Input: part model. Units: mm. Frame: model coordinates. A direction names the side the tool comes from. Round coordinates to 2 decimals unless told otherwise and drop trailing zeros. Loops run counter-clockwise (first coordinate to the right, second up) from the corner with the lowest first, then second, coordinate; pieces in that order, holes last. Notation, with made-up numbers: (-24.5, 70) -> (14.5, 70) arc R17 ccw to (14.5, 86) -> close; hole circle Ø5 at (45.25, 86.5). An arc over 180 degrees is marked (long way). One line per question, with ' | ' between items. Start each with the question number.
Q1. Cut plane B-B on z = 2.5. Return loops of the section in (x, y).
Q2. Access query for faces 1 (the face through (37, 44.45, 3)), 2 (the face through (-1.33, -5.59, 3.13)), 3 (the face through (0, 42, 3)). Directions: +Z, -Z, +X, -X, +Y, -Y. A direction counts if a zero-diameter tool reaches every point of the face in a straight line with its end or side. Return the directions, or none.
Q3. Cut plane D-D on y = 55. Return loops of the section in (x, z), and give its area (3 significant figures).
Q4. Material intervals for L1, parallel to X at y = 22.5, z = 4; L2, parallel to Y at x = 6.5, z = 6.25; L3, parallel to X at y = 52.5, z = 3, sorted ascending.
Q5. Cut plane C-C on x = 29. Return loops of the section in (y, z), and give its area (3 significant figures).
Q6. Contact query for flat-ended pins moving along their axis: P1, Ø3, axis at y = 46.5, z = 4, coming from the +X side; P2, Ø2, axis at x = 36, z = 4, coming from the +Y side; P3, Ø12, axis at x = 35.5, y = 43, coming from the -Z side; P4, Ø3, axis at x = 21.5, z = 2, coming from the +Y side. Output: stop coordinate, or through.
Q7. Cut plane A-A on y = 30.5. Return loops of the section in (x, z), and give its area (3 significant figures).
from build123d import *

# Parameters (mm, degrees)
BOSS_EXTRUDE1_DEPTH = 6.35
FILLET1_R           = 2.54


with BuildPart() as part:
    # Sketch1 → Boss-Extrude1 (new body)
    with BuildSketch(Plane.XY):
        Polygon((0, 0), (35.3568, 0), (35.3568, 44.45), (41.7068, 44.45), (41.7068, -6.35), (-2.0574, -6.35), (-2.0574, 82.55), (0, 82.55), align=None)
    extrude(amount=BOSS_EXTRUDE1_DEPTH)

    # Fillet1
    # the kernel refuses this fillet: 2.54 mm, written as the material it takes off along each edge
    with BuildSketch(Plane(origin=(41.7068, 44.45, -6.35), x_dir=(-1, 0, 0), z_dir=(0, 0, 1)), Plane(origin=(-2.0574, -6.35, -6.35), x_dir=(1, 0, 0), z_dir=(0, 0, 1)), Plane(origin=(41.7068, -6.35, -6.35), x_dir=(0, 1, 0), z_dir=(0, 0, 1))) as fillet1_piece_1:
        with BuildLine():
            CenterArc((FILLET1_R, FILLET1_R), FILLET1_R, 180, 90)
            Line((0, FILLET1_R), (-FILLET1_R * 0.02, FILLET1_R))
            Line((-FILLET1_R * 0.02, FILLET1_R), (-FILLET1_R * 0.02, -FILLET1_R * 0.02))
            Line((-FILLET1_R * 0.02, -FILLET1_R * 0.02), (FILLET1_R, -FILLET1_R * 0.02))
            Line((FILLET1_R, -FILLET1_R * 0.02), (FILLET1_R, 0))
        make_face()
    extrude(amount=19.05, mode=Mode.SUBTRACT)
    with BuildSketch(Plane(origin=(-2.0574, 82.55, -6.234328974), x_dir=(0, -1, 0), z_dir=(0, 0, 1))) as fillet1_piece_2:
        with BuildLine():
            CenterArc((2.493731589, 2.54), FILLET1_R, 190.952784199, 79.047215801)
            Line((0, 2.0574), (-0.049874632, 2.047748))
            ThreePointArc((-0.049874632, 2.047748), (-0.0508, 1.0287), (-0.0508, 0))
            Line((-0.0508, 0), (0, -0.0508))
            Line((0, -0.0508), (2.493731589, -0.0508))
            Line((2.493731589, -0.0508), (2.493731589, 0))
        make_face()
    extrude(amount=18.818657947, mode=Mode.SUBTRACT)


solid = part.part
Results:
1) outline: (-2.06, -3.81) arc R2.54 ccw to (0.48, -6.35) -> (39.17, -6.35) arc R2.54 ccw to (41.71, -3.81) -> (41.71, 41.91) arc R2.54 ccw to (39.17, 44.45) -> (35.36, 44.45) -> (35.36, 0) -> (0, 0) -> (0, 82.55) arc R2.54 ccw to (-2.06, 80.06) -> close
2) face 1: +Z, -Z, +X, +Y | face 2: +Z, -Z, -X, -Y | face 3: +Z, -Z, +Y
3) outline: (-2.06, 0) -> (0, 0) -> (0, 6.35) -> (-2.06, 6.35) -> close | area: 13.1 mm^2
4) L1: -2.06 to 0, 35.36 to 41.71 | L2: -6.35 to 0 | L3: -2.06 to 0
5) outline: (-6.35, 0) -> (0, 0) -> (0, 6.35) -> (-6.35, 6.35) -> close | area: 40.3 mm^2
6) P1: x = 0 | P2: y = 44.45 | P3: z = 0 | P4: y = 0
7) outline: (-2.06, 0) -> (0, 0) -> (0, 6.35) -> (-2.06, 6.35) -> close; (35.36, 0) -> (41.71, 0) -> (41.71, 6.35) -> (35.36, 6.35) -> close | area: 53.4 mm^2
